Part model, mm, in its own coordinate system. Round coordinates to 2 decimals unless told otherwise and drop trailing zeros. Loops run counter-clockwise (first coordinate to the right, second up) from the corner with the lowest first, then second, coordinate; pieces in that order, holes last.
from build123d import *

# Parameters (mm, degrees)
SKETCH1_R           = 1.25
BOSS_EXTRUDE1_DEPTH = 25
CUT_EXTRUDE1_DEPTH  = 2
CHAMFER1_SIZE       = 0.25


with BuildPart() as part:
    # Sketch1 → Boss-Extrude1 (new body)
    with BuildSketch(Plane(origin=(0, 0, 0), x_dir=(1, 0, 0), z_dir=(0, 1, 0))):
        Circle(SKETCH1_R)
    extrude(amount=BOSS_EXTRUDE1_DEPTH)

    # Sketch2 → Cut-Extrude1 (cut)
    with BuildSketch(Plane(origin=(0, 25, 0), x_dir=(1, 0, 0), z_dir=(0, 1, 0))):
        Polygon((0.866025404, 0), (0.433012702, 0.75), (-0.433012702, 0.75), (-0.866025404, 0), (-0.433012702, -0.75), (0.433012702, -0.75), align=None)
    extrude(amount=-CUT_EXTRUDE1_DEPTH, mode=Mode.SUBTRACT)

    # Chamfer1
    chamfer1_edges = [part.edges().sort_by_distance(p)[0] for p in [
        (-1.25, 25, 0),
    ]]
    chamfer(chamfer1_edges, length=CHAMFER1_SIZE)


solid = part.part
1) Mould opens along X. For faces 1 (the face through (0, 0, 0)), 2 (the face through (0, 24, 0.75)), 3 (the face through (0, 24, -0.75)), 4 (the face through (-0.27, 12.2, 1.22)) say: released by +X, released by -X, zero draft, split by the parting line, or undercut.
Values:
face 1: zero draft
face 2: undercut
face 3: undercut
face 4: split by the parting line
2) Slice it at A-A, the plane x = 0. Give the cut face in (y, z).
Values:
outline: (0, -1.25) - (24.75, -1.25) - (25, -1) - (25, -0.75) - (23, -0.75) - (23, 0.75) - (25, 0.75) - (25, 1) - (24.75, 1.25) - (0, 1.25) - close
3) Wall check: line 1 along X through (y, z) = (15, -0.9); line 2 along Z through (x, y) = (-1, 11.75); line 3 along Z through (x, y) = (-0.05, 20.25). Give the ranges that are in metal, low to high.
Values:
line 1: x = -0.87 to 0.87
line 2: z = -0.75 to 0.75
line 3: z = -1.25 to 1.25
4) Slice it at B-B, the plane y = 16. Give the cut face in (x, z).
Values:
outline: circle Ø2.5 at (0, 0)
